from build123d import *

# Parameters (mm, degrees)
SKETCH_1_W        = 80
SKETCH_1_H        = 80
EXTRUDE_1_DEPTH   = 2
CHAMFER_1_SIZE    = 2
HOLE_WIZARD_M81_D = 9


with BuildPart() as part:
    # Эскиз1 → Бобышка-Вытянуть1 (new body)
    with BuildSketch(Plane.XY):
        Rectangle(SKETCH_1_W, SKETCH_1_H)
    extrude(amount=EXTRUDE_1_DEPTH)

    # Фаска1
    chamfer_1_edges = [part.edges().sort_by_distance(p)[0] for p in [
        (40, -40, 1),
        (-40, -40, 1),
        (-40, 40, 1),
        (40, 40, 1),
    ]]
    chamfer(chamfer_1_edges, length=CHAMFER_1_SIZE)

    # Отверстие с зазором M81 (through all)
    with Locations(Plane.XY.offset(2)):
        with Locations((-20, 20), (20, 20), (-20, -20), (20, -20)):
            Hole(HOLE_WIZARD_M81_D / 2)


solid = part.part
CAD build for the part. Positions are in the model's coordinates, mm. Coordinates: 2 decimals unless noted, no trailing zeros. Write each loop counter-clockwise with the first axis right and the second up, starting at its lowest first coordinate (ties: lowest second). Pieces come first, ordered by that corner, then holes. Notation, with made-up numbers: M -38.5,78 L -14.5,78 A5 ccw -14.5,84 Z; hole C -30,-10 d4. An arc over 180 degrees is marked long. Answer as a JSON object with one key per item and string values. Group by question number.
1) Saw through at C-C (z = 1.15). Write the cut outline in (x, y).
2) Pin check, flat tips, straight feed: pin 1 Ø8 at (x, y) = (-20, 20) entering from +Z; pin 2 Ø2 at (x, y) = (6, -7.5) entering from -Z. Stop position of each tip, or through.
3) Saw through at A-A (x = -20). Write the cut outline in (y, z).
4) Wall check: line 1 (Y direction, x = 20, z = 1); line 2 (X direction, y = -22, z = 0.1); line 3 (Y direction, x = 16, z = 0.5). Give the ranges that are in metal, low to high. Write a range as from..to.
5) Mould opens along Y. For faces 1 (the face through (39, 39, 1)), 2 (the face through (-40, -1, 1)), 3 (the face through (-16.68, -16.96, 0.99)) say: +Y half, -Y half, draft (parallel to the pull), parting line (faces both ways), or undercut.
Values follow:
{
 "1": {"outline": "M -40,-38 L -38,-40 L 38,-40 L 40,-38 L 40,38 L 38,40 L -38,40 L -40,38 Z; hole C -20,-20 d9; hole C -20,20 d9; hole C 20,-20 d9; hole C 20,20 d9"},
 "2": {"pin 1": "passes through", "pin 2": "stops at z = 0"},
 "3": {"outline": "M -40,0 L -24.5,0 L -24.5,2 L -40,2 Z; M -15.5,0 L 15.5,0 L 15.5,2 L -15.5,2 Z; M 24.5,0 L 40,0 L 40,2 L 24.5,2 Z"},
 "4": {"line 1": "y = -40..-24.5, -15.5..15.5, 24.5..40", "line 2": "x = -40..-24.03, -15.97..15.97, 24.03..40", "line 3": "y = -40..-22.06, -17.94..17.94, 22.06..40"},
 "5": {"face 1": "+Y half", "face 2": "draft", "face 3": "undercut"}
}
